```python
from build123d import *

# Parameters (mm, degrees)
F0_W     = 111.76
F0_H     = 73.66
F1_DEPTH = 86.868
F2_W     = 19.05
F2_H     = 19.05
F2_W_2   = 13.97
F2_H_2   = 13.97
F2_W_3   = 63.5
F3_DEPTH = 15.875
F4_R     = 5.08
F5_R     = 5.08


with BuildPart() as f1:
    # F0 (on Top) → F1 (new body)
    with BuildSketch(Plane.XY):
        Rectangle(F0_W, F0_H)
    extrude(amount=F1_DEPTH)

    # F2 (on face) → F3 (cut)
    with BuildSketch(Plane.XY.offset(86.868)):
        with Locations((-46.355, -27.305)):
            Rectangle(F2_W, F2_H)
        with Locations((-46.355, -27.305)):
            Rectangle(F2_W_2, F2_H_2, mode=Mode.SUBTRACT)
        with Locations((0, -27.305)):
            Rectangle(F2_W_3, F2_H)
        with Locations((46.355, -27.305)):
            Rectangle(F2_W, F2_H)
        with Locations((46.355, -27.305)):
            Rectangle(F2_W_2, F2_H_2, mode=Mode.SUBTRACT)
    extrude(amount=-F3_DEPTH, mode=Mode.SUBTRACT)

    # F4
    f4_edges = [f1.edges().sort_by_distance(p)[0] for p in [
        (34.29, -36.83, 86.868),
        (-34.29, -36.83, 86.868),
        (55.88, 9.525, 86.868),
        (0, 36.83, 86.868),
        (-55.88, 9.525, 86.868),
        (-55.88, -36.83, 35.4965),
        (55.88, -36.83, 35.4965),
        (55.88, 36.83, 43.434),
        (-55.88, 36.83, 43.434),
    ]]
    fillet(f4_edges, radius=F4_R)

    # F5
    f5_edges = [f1.edges().sort_by_distance(p)[0] for p in [
        (55.88, 0, 0),
        (54.392102, -35.342102, 0),
        (54.392102, 35.342102, 0),
        (0, -36.83, 0),
        (0, 36.83, 0),
        (-54.392102, -35.342102, 0),
        (-54.392102, 35.342102, 0),
        (-55.88, 0, 0),
    ]]
    fillet(f5_edges, radius=F5_R)


solid = f1.part
```
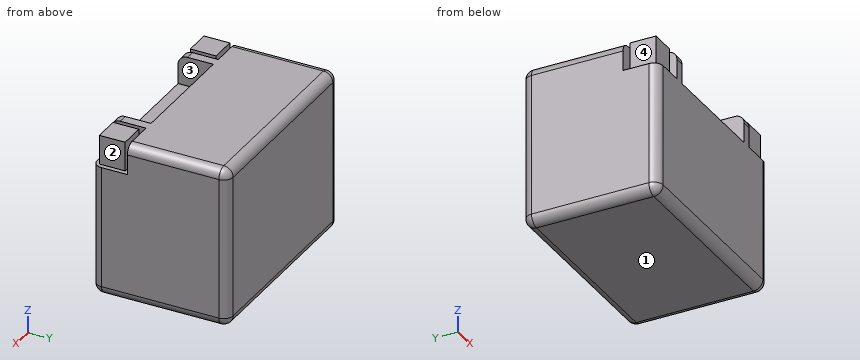
CAD build for the part. Positions are in the model's coordinates, mm. Face numbers are marked on the shaded views. A direction names the side the tool comes from. Round coordinates to 2 decimals unless told otherwise and drop trailing zeros. Write each loop counter-clockwise with the first axis right and the second up, starting at its lowest first coordinate (ties: lowest second). Pieces come first, ordered by that corner, then holes. Notation, with made-up numbers: (17.5, 72.25) - (53.5, 72.25) arc R37 cw to (53.5, 111.25) - close; hole circle Ø10 at (-1.75, 40). An arc over 180 degrees is marked (long way). Return JSON: item names as keys, results as strings. Group by question number.
Item 1: Probe probe 1 along Y at (x, z) = (7, 79); probe 2 along Z at (x, y) = (-21.5, -22); probe 3 along X at (y, z) = (32, 82.5). List the from-to ranges inside material, lowest first.
Item 2: Band-saw the part on A-A on z = 77.5. List the corners of the cut face in (x, y), plus the area to 3 significant figures.
Item 3: Band-saw the part on C-C on x = -5.5. List the corners of the cut face in (y, z).
Item 4: Flat gauge pins, fed straight in: pin 1 Ø7 at (y, z) = (-29.5, 75.5) entering from -X; pin 2 Ø8 at (y, z) = (-31.5, 79) entering from +X; pin 3 Ø5 at (x, z) = (-47.5, 78) entering from -Y. Where does each tip first touch, or does it go through?
Item 5: 3-axis set-ups, long thin cutter, end or side, ignore diameter. For the marked faces 1, 2, 3 and 4: which of +Z, -Z, +X, -X, +Y, -Y reach the whole face in a straight line?
Item 6: Band-saw the part on B-B on x = 44. List the corners of the cut face in (y, z), plus the area to 3 significant figures.
Resolved:
{
 "1": {"probe 1": "y = -17.78 to 36.83", "probe 2": "z = 0 to 70.99", "probe 3": "x = -55.82 to 55.82"},
 "2": {"outline": "(-55.88, -17.78) - (-36.83, -17.78) - (-36.83, -36.83) - (-31.75, -36.83) - (-31.75, -17.78) - (31.75, -17.78) - (31.75, -36.83) - (36.83, -36.83) - (36.83, -17.78) - (55.88, -17.78) - (55.88, 31.75) arc R5.08 ccw to (50.8, 36.83) - (-50.8, 36.83) arc R5.08 ccw to (-55.88, 31.75) - close; (-53.34, -34.29) - (-39.37, -34.29) - (-39.37, -20.32) - (-53.34, -20.32) - close; (39.37, -34.29) - (53.34, -34.29) - (53.34, -20.32) - (39.37, -20.32) - close", "area": "6,680 mm²"},
 "3": {"outline": "(-36.83, 5.08) arc R5.08 ccw to (-31.75, 0) - (31.75, 0) arc R5.08 ccw to (36.83, 5.08) - (36.83, 81.79) arc R5.08 ccw to (31.75, 86.87) - (-17.78, 86.87) - (-17.78, 70.99) - (-36.83, 70.99) - close"},
 "4": {"pin 1": "stops at x = -53.34", "pin 2": "stops at x = 53.34", "pin 3": "stops at y = -34.29"},
 "5": {"face 1": "-Z, +X, -X, +Y, -Y", "face 2": "+Z, +X, -Y", "face 3": "+Z, -Y", "face 4": "+Z, -X, -Y"},
 "6": {"outline": "(-36.83, 5.08) arc R5.08 ccw to (-31.75, 0) - (31.75, 0) arc R5.08 ccw to (36.83, 5.08) - (36.83, 81.79) arc R5.08 ccw to (31.75, 86.87) - (-17.78, 86.87) - (-17.78, 70.99) - (-20.32, 70.99) - (-20.32, 86.87) - (-34.29, 86.87) - (-34.29, 70.99) - (-36.83, 70.99) - close", "area": "6,300 mm²"}
}
